Check sheet for the modelled part. Datum: model origin and axes. Units: mm. Round coordinates to 2 decimals unless told otherwise and drop trailing zeros. Order: outer loops, then holes, each group sorted by start corner. A loop starts at its lowest first (then second) coordinate and runs counter-clockwise, first axis right, second up.
Autodesk Inventor part; units mm, degrees
ref_plane "YZ Plane" through (0, 0, 0) normal (1, 0, 0) x (0, 1, 0)
ref_plane "XZ Plane" through (0, 0, 0) normal (0, 1, 0) x (-1, 0, 0)
ref_plane "XY Plane" through (0, 0, 0) normal (0, 0, 1) x (1, 0, 0)
sketch "Sketch1" plane through (0, 0, 0) normal (1, 0, 0) x (0, 1, 0)
  line L0 (0, 0) -> (25.4, 0)
  line L1 (25.4, 0) -> (25.4, -25.4)
  line L2 (25.4, -25.4) -> (0, -25.4)
  line L3 (0, -25.4) -> (0, 0)
  line L4 (3.175, -3.175) -> (22.225, -3.175)
  line L5 (22.225, -3.175) -> (22.225, -22.225)
  line L6 (22.225, -22.225) -> (3.175, -22.225)
  line L7 (3.175, -22.225) -> (3.175, -3.175)
  dimension "d0" = 25.4
  dimension "d1" = 25.4
  dimension "d2" = 19.05
  dimension "d3" = 19.05
  dimension "d4" = 3.175
  dimension "d5" = 3.175
extrude "Extrusion1" add sketch "Sketch1" along normal blind 546.1
sketch "Sketch2" plane through (0, 25.4, 0) normal (0, 1, 0) x (1, 0, 0)
  line L0 (0, 0) -> (0, 25.4)
  line L1 (0, 0) -> (546.1, 0)
  line L2 (546.1, 25.4) -> (546.1, 0)
  line L3 (0, 25.4) -> (546.1, 25.4)
  point P0 (12.7, 15.875)
  point P1 (533.4, 15.875)
  dimension "d8" = 15.875
  dimension "d9" = 12.7
  dimension "d10" = 12.7
  dimension "d11" = 15.875
hole "Hole1" at (12.7, 25.4, -15.875) at (533.4, 25.4, -15.875) direction (0, -1, 0) diameter 6.35 end through all
sketch "Sketch3" plane through (0, 25.4, 0) normal (0, 1, 0) x (1, 0, 0)
  circle A0 centre (12.7, 15.875) radius 3.175
  circle A1 centre (533.4, 15.875) radius 3.175
  line L0 (0, 0) -> (0, 25.4)
  line L1 (0, 0) -> (546.1, 0)
  line L2 (546.1, 25.4) -> (546.1, 0)
  line L3 (0, 25.4) -> (546.1, 25.4)
  point P0 (38.1, 15.875)
  point P1 (508, 15.875)
  point P2 (296.8625, 15.875)
  point P3 (249.2375, 15.875)
  dimension "d19" = 38.1
  dimension "d20" = 38.1
  dimension "d21" = 15.875
  dimension "d22" = 15.875
  dimension "d30" = 15.875
  dimension "d31" = 249.2375
  dimension "d39" = 249.2375
  dimension "d40" = 15.875
hole "Hole4" at (38.1, 25.4, -15.875) at (508, 25.4, -15.875) at (296.8625, 25.4, -15.875) at (249.2375, 25.4, -15.875) direction (0, -1, 0) diameter 6.35 end through all
properties part number "mounting block medium" material "Aluminum 6061"
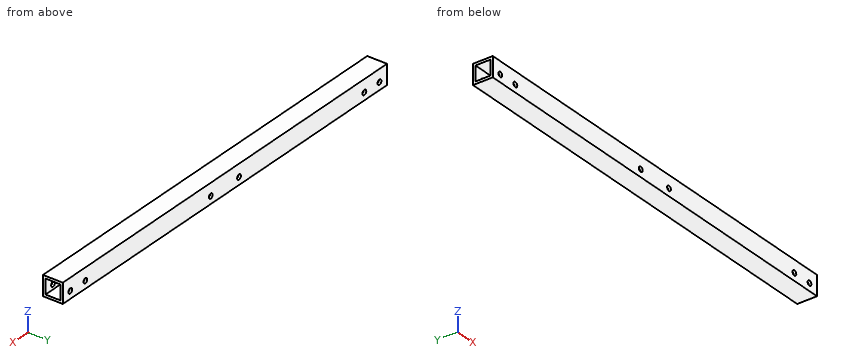
Item 1: Sectioned sample at B-B (y = 8.75). Record the cut outline in (x, z) (3 decimals).
Answer:
outline: (0, -25.4) - (546.1, -25.4) - (546.1, -22.225) - (0, -22.225) - close; (0, -3.175) - (546.1, -3.175) - (546.1, 0) - (0, 0) - close
Item 2: Sectioned sample at A-A (x = 334). Record the cut outline in (y, z) (3 decimals), and give its area (3 significant figures).
Answer:
outline: (0, -25.4) - (25.4, -25.4) - (25.4, 0) - (0, 0) - close; hole (3.175, -22.225) - (22.225, -22.225) - (22.225, -3.175) - (3.175, -3.175) - close
area: 282 mm2
Item 3: Scan lines: line 1 along Y through (x, z) = (434, -17) (3 decimals); line 2 along Z through (x, y) = (400.5, 18) (3 decimals); line 3 along Z through (x, y) = (533.4, 2.25). Record each from-to range of solid material in increasing order.
Answer:
line 1: y = 0 to 3.175, 22.225 to 25.4
line 2: z = -25.4 to -22.225, -3.175 to 0
line 3: z = -25.4 to -19.05, -12.7 to 0
